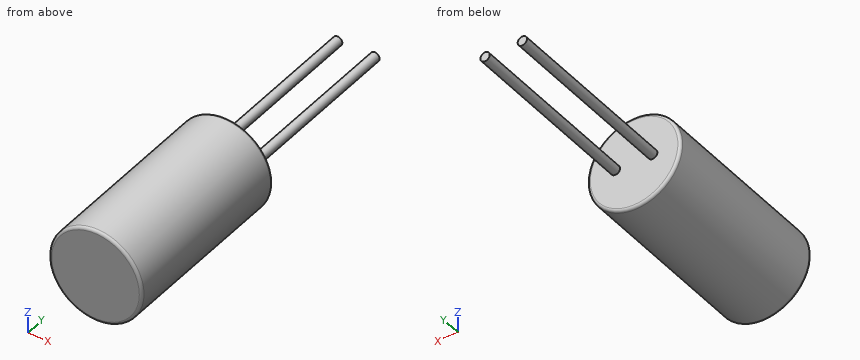
```python
from build123d import *

# Parameters (mm, degrees)
SKETCH1_R           = 5
BOSS_EXTRUDE1_DEPTH = 20
SKETCH2_R           = 0.5
BOSS_EXTRUDE2_DEPTH = 20
FILLET1_R           = 0.3


with BuildPart() as part:
    # Sketch1 → Boss-Extrude1 (new body)
    with BuildSketch(Plane(origin=(0, 0, 0), x_dir=(1, 0, 0), z_dir=(0, 1, 0))):
        Circle(SKETCH1_R)
    extrude(amount=BOSS_EXTRUDE1_DEPTH)

    # Sketch2 → Boss-Extrude2 (add)
    with BuildSketch(Plane(origin=(0, 20, 0), x_dir=(1, 0, 0), z_dir=(0, 1, 0))):
        with Locations((-2, 0)):
            Circle(SKETCH2_R)
        with Locations((2, 0)):
            Circle(SKETCH2_R)
    extrude(amount=BOSS_EXTRUDE2_DEPTH)

    # Fillet1
    fillet1_edges = [part.edges().sort_by_distance(p)[0] for p in [
        (-5, 0, 0),
        (-5, 20, 0),
    ]]
    fillet(fillet1_edges, radius=FILLET1_R)


solid = part.part
```
Check sheet for the modelled part. Datum: model origin and axes. Units: mm. Round coordinates to 2 decimals unless told otherwise and drop trailing zeros. Order: outer loops, then holes, each group sorted by start corner. A loop starts at its lowest first (then second) coordinate and runs counter-clockwise, first axis right, second up. Notation, with made-up numbers: (-33.5, 26.25) - (-18.5, 26.25) arc R25 ccw to (-18.5, 61.25) - close; hole circle Ø10 at (5.25, 63). An arc over 180 degrees is marked (long way). Write item = value, one per line.
Q1. Go/stop test with a flat-tipped pin: pin 1 (4 mm diameter, centred on y = 35, z = -3, fed in from -X). Record where the tip stops, or that it passes through.
Computed:
pin_1 = through
Q2. Section check C-C (z = 0). Record the boundary of the cut face in (x, y), and give its area (3 significant figures).
Computed:
outline = (-5, 0.3) arc R0.3 ccw to (-4.7, 0) - (4.7, 0) arc R0.3 ccw to (5, 0.3) - (5, 19.7) arc R0.3 ccw to (4.7, 20) - (2.5, 20) - (2.5, 40) - (1.5, 40) - (1.5, 20) - (-1.5, 20) - (-1.5, 40) - (-2.5, 40) - (-2.5, 20) - (-4.7, 20) arc R0.3 ccw to (-5, 19.7) - close
area = 240 mm^2
Q3. Section check A-A (x = 0). Record the boundary of the cut face in (y, z), and give its area (3 significant figures).
Computed:
outline = (0, -4.7) arc R0.3 ccw to (0.3, -5) - (19.7, -5) arc R0.3 ccw to (20, -4.7) - (20, 4.7) arc R0.3 ccw to (19.7, 5) - (0.3, 5) arc R0.3 ccw to (0, 4.7) - close
area = 200 mm^2
Q4. Section check D-D (y = 9). Record the boundary of the cut face in (x, z), and give its area (3 significant figures).
Computed:
outline = circle Ø10 at (0, 0)
area = 78.5 mm^2
Q5. Section check B-B (y = 27). Record the boundary of the cut face in (x, z).
Computed:
outline = circle Ø1 at (-2, 0); circle Ø1 at (2, 0)
Q6. Thickness scan on line 1 along Y through (x, z) = (-0.25, -2.5); line 2 along X through (y, z) = (5.5, -0.25); line 3 along X through (y, z) = (8.5, -3.75). Record the ranges inside material, lowest first.
Computed:
line_1 = 0 to 20
line_2 = -4.99 to 4.99
line_3 = -3.31 to 3.31
